```python
from build123d import *

# Parameters (mm, degrees)
CYLINDER027_R             = 3.25
CYLINDER027_DEPTH         = 10
ARRAY009_X_COUNT          = 2
ARRAY009_X_PITCH          = 174
BOX051_W                  = 138
BOX051_H                  = 108
BOX051_DEPTH              = 37
BOX049_W                  = 152
BOX049_H                  = 145
BOX049_DEPTH              = 10
BOX048_W                  = 190
BOX048_H                  = 145
BOX048_DEPTH              = 10
BOX050_W                  = 149
BOX050_H                  = 118
BOX050_DEPTH              = 20
FILLET001_R               = 10
FILLET002_R               = 8
FILLET003_R               = 5
FILLET003_PLACEMENT_ANGLE = 180


with BuildPart() as array009:
    # Cylinder027 → Cylinder027 (new body)
    with BuildSketch(Plane(origin=(8, 75, 0), x_dir=(1, 0, 0), z_dir=(0, 0, 1))):
        Circle(CYLINDER027_R)
    extrude(amount=CYLINDER027_DEPTH)

    # Array009 X: Array009 ×2


with BuildPart() as array009_1:
    add(array009.part)
    with Locations(*[(i * ARRAY009_X_PITCH, 0, 0) for i in range(1, ARRAY009_X_COUNT)]):
        add(array009.part)


with BuildPart() as array009_2:
    # Array009 placement: moved
    add(array009_1.part.moved(Location((-74, -75, -54))))


with BuildPart() as cubo038:
    # Box051 → Box051 (new body)
    with BuildSketch(Plane(origin=(26, 19, -4), x_dir=(1, 0, 0), z_dir=(0, 0, 1))):
        with Locations((69, 54)):
            Rectangle(BOX051_W, BOX051_H)
    extrude(amount=BOX051_DEPTH)


with BuildPart() as cubo036:
    # Box049 → Box049 (new body)
    with BuildSketch(Plane(origin=(19, 0, 3), x_dir=(1, 0, 0), z_dir=(0, 0, 1))):
        with Locations((76, 72.5)):
            Rectangle(BOX049_W, BOX049_H)
    extrude(amount=BOX049_DEPTH)


with BuildPart() as cubo035:
    # Box048 → Box048 (new body)
    with BuildSketch(Plane.XY):
        with Locations((95, 72.5)):
            Rectangle(BOX048_W, BOX048_H)
    extrude(amount=BOX048_DEPTH)


with BuildPart() as obj1:
    # Box050 → Box050 (new body)
    with BuildSketch(Plane(origin=(20.5, 13.5, 3), x_dir=(1, 0, 0), z_dir=(0, 0, 1))):
        with Locations((74.5, 59)):
            Rectangle(BOX050_W, BOX050_H)
    extrude(amount=BOX050_DEPTH)

    # Fusion026: union Cubo036, Cubo035
    add(cubo036.part)
    add(cubo035.part)

    # Cut035: cut Cubo038
    add(cubo038.part, mode=Mode.SUBTRACT)

    # Fillet001
    fillet001_edges = [obj1.edges().sort_by_distance(p)[0] for p in [
        (164, 19, 11.5),
        (26, 19, 11.5),
        (164, 127, 11.5),
        (26, 127, 11.5),
    ]]
    fillet(fillet001_edges, radius=FILLET001_R)

    # Fillet002
    fillet002_edges = [obj1.edges().sort_by_distance(p)[0] for p in [
        (20.5, 13.5, 18),
        (20.5, 131.5, 18),
        (169.5, 131.5, 18),
        (169.5, 13.5, 18),
    ]]
    fillet(fillet002_edges, radius=FILLET002_R)

    # Fillet003
    fillet003_edges = [obj1.edges().sort_by_distance(p)[0] for p in [
        (20.5, 72.5, 23),
        (22.843146, 15.843146, 23),
        (22.843146, 129.156854, 23),
        (95, 13.5, 23),
        (95, 131.5, 23),
        (167.156854, 15.843146, 23),
        (167.156854, 129.156854, 23),
        (169.5, 72.5, 23),
    ]]
    fillet(fillet003_edges, radius=FILLET003_R)


with BuildPart() as obj1_1:
    # Fillet003 placement: moved
    add(obj1.part.moved(Location((-72, 71, -44))).rotate(Axis((-72, 71, -44), (1, 0, 0)), FILLET003_PLACEMENT_ANGLE))

    # Cut036: cut Array009
    add(array009_2.part, mode=Mode.SUBTRACT)


solid = obj1_1.part
```
Source: CAD feature listing. Evaluate the final solid. Frame: model axes, mm. A direction names the side the tool comes from. Round coordinates to 2 decimals unless told otherwise and drop trailing zeros. Order: outer loops, then holes, each group sorted by start corner. A loop starts at its lowest first (then second) coordinate and runs counter-clockwise, first axis right, second up. Notation, with made-up numbers: (19, 5.5) -> (63, 5.5) arc R16 ccw to (63, 25.5) -> close; hole circle Ø10 at (-12.5, 16.25). An arc over 180 degrees is marked (long way). Use CSV: the item, a comma, the result in double quotes.
(1) Ray query, L1, parallel to X at y = 21, z = -61.5; L2, parallel to Y at x = 71, z = -60.25; L3, parallel to Y at x = -66, z = -51.5. Return the intervals inside material, ascending.
Report:
L1,"-51.5 to -46, 92 to 97.5"
L2,"-60.5 to -56, 52 to 57.5"
L3,"-74 to -3.25, 3.25 to 71"
(2) Section B-B on y = 0. Return the cut outline in (x, z).
Report:
outline,"(-72, -54) -> (-69.25, -54) -> (-69.25, -44) -> (-72, -44) -> close; (-62.75, -54) -> (-53, -54) -> (-53, -57) -> (-51.5, -57) -> (-51.5, -62) arc R5 ccw to (-46.5, -67) -> (-46, -67) -> (-46, -44) -> (-62.75, -44) -> close; (92, -67) -> (92.5, -67) arc R5 ccw to (97.5, -62) -> (97.5, -57) -> (99, -57) -> (99, -54) -> (104.75, -54) -> (104.75, -44) -> (92, -44) -> close; (111.25, -54) -> (118, -54) -> (118, -44) -> (111.25, -44) -> close"
(3) Pull-direction query (Y, two-part tool) for faces 5 (the face through (-49.219, -58.094, -59.535)), 6 (the face through (-51.5, -1, -59)), 7 (the face through (-43.15, 48.99, -55.66)), 8 (the face through (104.753, 0.143, -49.07)); classes: +Y half, -Y half, draft (parallel to the pull), parting line (faces both ways), or undercut.
Report:
face 5,"-Y half"
face 6,"draft"
face 7,"undercut"
face 8,"undercut"
(4) Access query for faces 1 (the face through (22, -60.5, -59)), 2 (the face through (89.15, -52.99, -55.66)), 3 (the face through (95.094, -58.219, -59.535)), 4 (the face through (22, 57.5, -59)). Directions: +Z, -Z, +X, -X, +Y, -Y. A direction counts if a zero-diameter tool reaches every point of the face in a straight line with its end or side. Return the directions, or none.
Report:
face 1,"-Z, +X, -X, -Y"
face 2,"+Z, -Z"
face 3,"-Z, +X, -Y"
face 4,"-Z, +X, -X, +Y"
(5) First-contact query: pin 1 Ø4 at (y, z) = (3.5, -54.5) entering from -X; pin 2 Ø4 at (y, z) = (-7.5, -59.5) entering from -X; pin 3 Ø5.5 at (x, z) = (27, -60) entering from +Y; pin 4 Ø4 at (x, z) = (47.5, -60.5) entering from -Y. Flat tips, straight axial feed; report the tip coordinate or a pass-through.
Report:
pin 1,"x = -72"
pin 2,"x = -51.5"
pin 3,"y = 57.5"
pin 4,"y = -60.5"
(6) Section C-C on y = -32.5. Return the cut outline in (x, z).
Report:
outline,"(-72, -54) -> (-53, -54) -> (-53, -57) -> (-51.5, -57) -> (-51.5, -62) arc R5 ccw to (-46.5, -67) -> (-46, -67) -> (-46, -44) -> (-72, -44) -> close; (92, -67) -> (92.5, -67) arc R5 ccw to (97.5, -62) -> (97.5, -57) -> (99, -57) -> (99, -54) -> (118, -54) -> (118, -44) -> (92, -44) -> close"
(7) Section A-A on x = -66. Return the cut outline in (y, z), and give its area (4 significant figures).
Report:
outline,"(-74, -54) -> (-3.25, -54) -> (-3.25, -44) -> (-74, -44) -> close; (3.25, -54) -> (71, -54) -> (71, -44) -> (3.25, -44) -> close"
area,"1,385 mm^2"
